Verification items for the finished model (mm, model axes). Face numbers are marked on the shaded views. Round coordinates to 2 decimals unless told otherwise and drop trailing zeros. Write each loop counter-clockwise with the first axis right and the second up, starting at its lowest first coordinate (ties: lowest second). Pieces come first, ordered by that corner, then holes. Notation, with made-up numbers: (83, -34.75) - (89, -34.75) arc R24 cw to (89, -13.75) - close; hole circle Ø8 at (-14.75, 18). An arc over 180 degrees is marked (long way). Answer as a JSON object with one key per item and string values.
Autodesk Inventor part; units mm, degrees
ref_plane "Work Plane1" through (2.75, 0, 0) normal (0, -1, 0) x (1, 0, 0)
ref_plane "YZ Plane" through (0, 0, 0) normal (1, 0, 0) x (0, 1, 0)
ref_plane "XZ Plane" through (0, 0, 0) normal (0, 1, 0) x (-1, 0, 0)
sketch "Skizze1" plane through (0, 0, 0) normal (0, 0, 1) x (1, 0, 0)
  line L0 (20, 4) -> (20, 0)
  line L1 (-8, 0) -> (20, 0)
  line L2 (-13.6, 0) -> (25.6, 0)
  line L3 (0, 4.8) -> (0, -0.8)
  line L4 (-8, 4) -> (-8, 0)
  line L5 (2, 4) -> (2, 0) construction
  line L6 (-13.6, 0) -> (25.6, 0)
  line L7 (-8, 4) -> (20, 4)
  dimension "d4" = 8
  dimension "d5" = 20
  dimension "d6" = 18
  dimension "d13" = 8
revolve "Körper" add sketch "Skizze1" angle 360 about axis through (-8, 0, 0) along (1, 0, 0)
thread "Gewinde1"
thread "Gewinde2"
chamfer "Fase1" distance 0.7678 distance2 0.7668 1 edges at (20, -4, 0) measured on face at (20, -0.0467, 2.2623)
chamfer "Fase2" distance 1.251 distance2 0.7668 1 edges at (-8, -4, 0) measured on face at (10.1555, 3.987, -0.3219)
ref_plane "Work Plane1" through (2.75, 0, 0) normal (0, -1, 0) x (1, 0, 0)
equation "\"d4\" = KOH"
equation "\"d5\" = NLG"
equation "\"d6\" = GEL"
equation "\"d13\" = GD"
equation "\"d1\" = KOH"
equation "\"d7\" = GEL + GAL"
equation "\"d10\" = -0.5 * SPD + 0.5 * GD"
equation "\"d12\" = -0.5 * SPD + 0.5 * GD"
equation "\"NLG\" = 20"
equation "\"GEL\" = 18"
equation "\"GAL\" = 0.61345 * PTC"
equation "\"SPD\" = NND - 1.2269 * PTC"
equation "\"d0\" = GD"
equation "\"GUL\" = 0.61345 * PTC"
equation "\"KOH\" = NND"
equation "\"GD\" = NND"
equation "\"BDM\" = NND"
equation "\"GUL1\" = 1.25"
equation "\"GAL1\" = 1.25"
equation "\"d80\" = -GUL - GEL"
equation "\"d86\" = -KOH + GUL1"
equation "\"PTC\" = 1.25"
equation "\"THREADDIA\" = 8"
equation "\"TOA\" = 30deg"
equation "\"NND\" = 8"
equation "\"GD1\" = THREADDIA - 1.2269 * PTC"
properties part number "CSN 02 1174 - A M8 x 20" material "Stahl, weich"
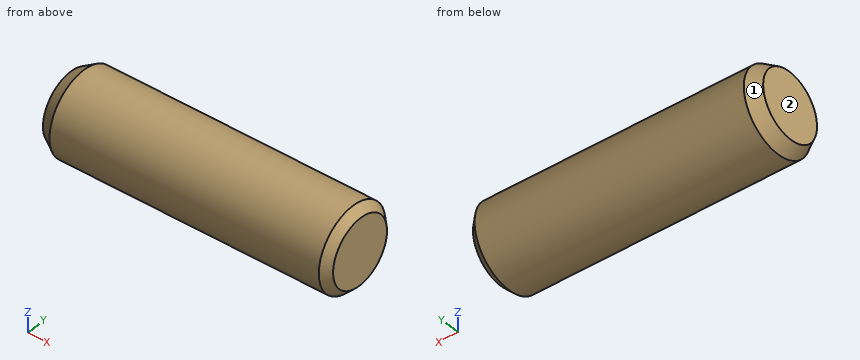
Q1. Gauge pin test, flat end, axial feed: P1, Ø2, axis at x = 6, y = -3, coming from the -Z side. Record the tip position at first contact, or that the pin passes through.
Geometry check:
{"P1": "stops at z = -3.46"}
Q2. Release check for a two-part mould opening along Y. For the marked faces 1 and 2 record: released by +Y, released by -Y, zero draft, split by the parting line, or undercut.
Geometry check:
{"face 1": "split by the parting line", "face 2": "zero draft"}
Q3. Material ranges on line 1 along Y through (x, z) = (10.75, 2.25); line 2 along Y through (x, z) = (13.75, -3); line 3 along Z through (x, y) = (5.75, -2.75), recorded low to high. Write a range as [from, to].
Geometry check:
{"line 1": "y = [-3.31, 3.31]", "line 2": "y = [-2.65, 2.65]", "line 3": "z = [-2.9, 2.9]"}
Q4. Section check A-A, the plane x = 7. Record the cut outline in (y, z).
Geometry check:
{"outline": "circle Ø8 at (0, 0)"}
